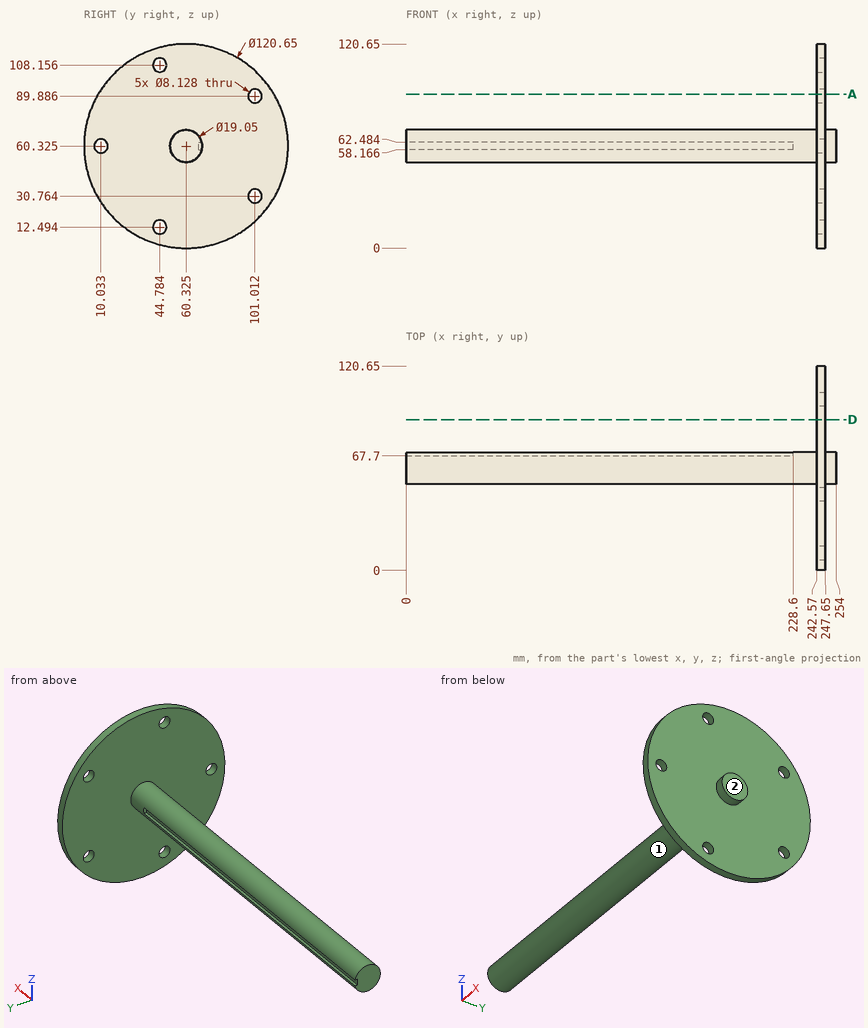
Verification items for this drawing (mm, ordinates from the low corner). A direction names the side the tool comes from. Coordinates: 2 decimals unless noted, no trailing zeros. Loops run counter-clockwise (first coordinate to the right, second up) from the corner with the lowest first, then second, coordinate; pieces in that order, holes last. Notation, with made-up numbers: (-13, 43.5) - (15, 43.5) arc R8 cw to (15, 51.5) - close; hole circle Ø1 at (37, 64). An arc over 180 degrees is marked (long way). Answer as a JSON object with one key per item and string values.
(1) Go/stop test with flat-tipped pins: pin 1 Ø12 at (y, z) = (41, 71) entering from -X; pin 2 Ø1.5 at (y, z) = (37, 26) entering from +X; pin 3 Ø1.1 at (y, z) = (68.5, 59.5) entering from -X. Record where each tip stops, or that it passes through.
Response:
{"pin 1": "stops at x = 242.57", "pin 2": "stops at x = 247.65", "pin 3": "stops at x = 228.6"}
(2) Access from +Z, -Z, +X, -X, +Y, -Y to the whole of each face (thin tool, end or side, straight path). Record for the marked faces 1 and 2.
Response:
{"face 1": "-X", "face 2": "+Z, -Z, +X, +Y, -Y"}
(3) Cross-section at A-A, the plane z = 91. Record the boundary of the cut face in (x, y).
Response:
{"outline": "(242.57, 8.38) - (247.65, 8.38) - (247.65, 97.1) - (242.57, 97.1) - close; (242.57, 104.92) - (247.65, 104.92) - (247.65, 112.27) - (242.57, 112.27) - close"}
(4) Scan lines: line 1 along X through (y, z) = (52.5, 29.5); line 2 along Y through (x, z) = (232, 61) (1 decimal); line 3 along Z through (x, y) = (218.5, 65) (1 decimal). Record each from-to range of solid material in increasing order.
Response:
{"line 1": "x = 242.57 to 247.65", "line 2": "y = 50.8 to 69.8", "line 3": "z = 52 to 68.6"}
(5) Cross-section at D-D, the plane y = 89. Record the boundary of the cut face in (x, z), then the cut area to 3 significant figures.
Response:
{"outline": "(242.57, 7.25) - (247.65, 7.25) - (247.65, 113.4) - (242.57, 113.4) - close", "area": "539 mm²"}
